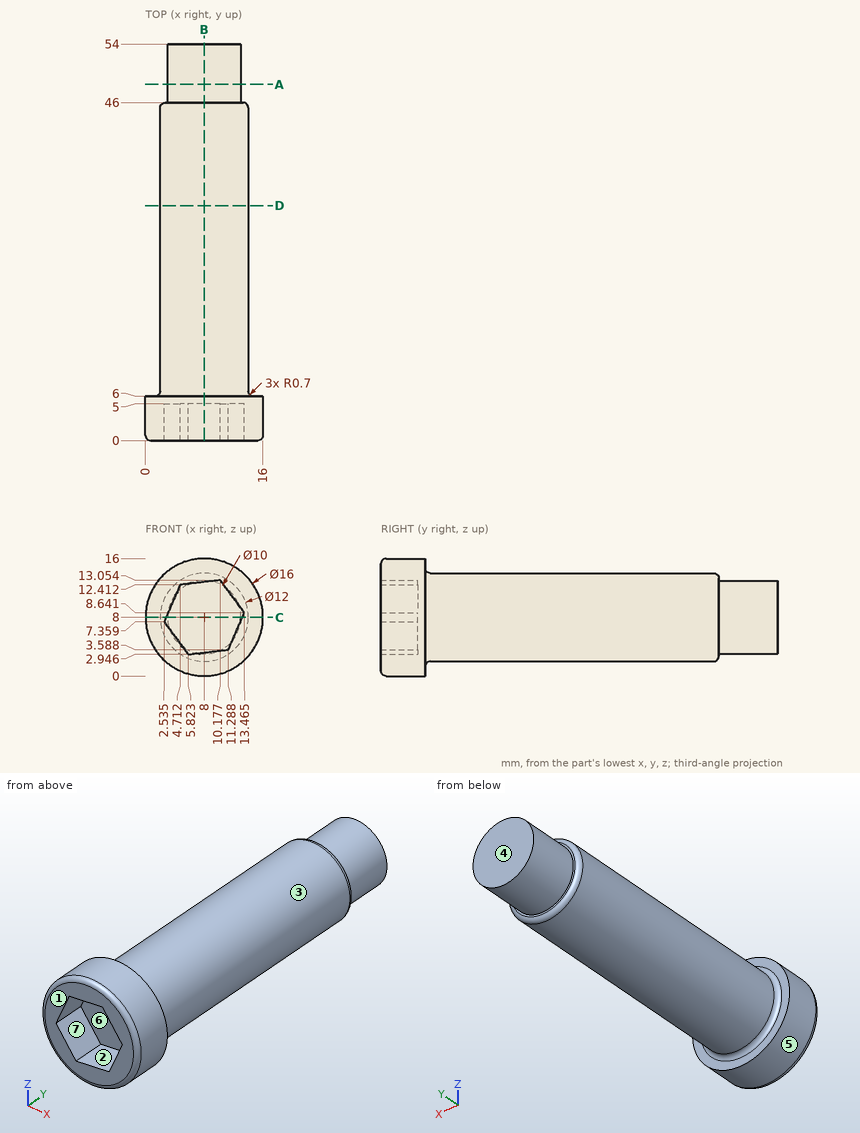
Could you check a few things on this drawing? It's one solid part, dimensions in mm from its lowest x, y, z. A direction names the side the tool comes from. Coordinates: 2 decimals unless noted, no trailing zeros. Order: outer loops, then holes, each group sorted by start corner. A loop starts at its lowest first (then second) coordinate and runs counter-clockwise, first axis right, second up. Notation, with made-up numbers: (39.25, 21.5) - (68.25, 21.5) arc R18 ccw to (68.25, 45.5) - close; hole circle Ø8 at (62.25, -11.5). An arc over 180 degrees is marked (long way). Answer as a JSON object with one key per item and string values. Group by question number.
Q1. Imagine slicing it at A-A (y = 48.5). Please give me the cut outline in (x, z).
Q2. Imagine slicing it at B-B (x = 8). Please give me the cut outline in (y, z).
Q3. On a 3-axis mill with a long thin cutter (end or side, diameter ignored), from which of +Z, -Z, +X, -X, +Y, -Y can I reach the whole of each face in a straight line? I mean the marked faces 1, 2 and 3. Say none if no direction works.
Q4. Imagine slicing it at D-D (y = 32). Please give me the cut outline in (x, z), and give its area (3 significant figures).
Q5. Will these pins go through, and if not, where does the flat tip stop? P1, Ø1.5, axis at y = 26, z = 8.5, coming from the -X side; P2, Ø2, axis at x = 10.5, y = 13.5, coming from the +Z side; P3, Ø3, axis at x = 3, y = 46.5, coming from the -Z side (1 decimal).
Q6. Imagine slicing it at C-C (z = 8). Please give me the cut outline in (x, y).
Q7. We'd pull the mould along X, two halves only. Please class the marked faces 4, 5, 6 and 7: +X half, -X half, draft (parallel to the pull), parting line (faces both ways), or undercut.
Q8. I need wall thicknesses on line 1 (Y direction, x = 5.75, z = 4.75); line 2 (Y direction, x = 12.25, z = 4.75); line 3 (Z direction, x = 7.75, y = 14) (1 decimal). Which ranges of each line are inside material? Lowest first, please. Write a range as from..to.
Determined:
{
 "1": {"outline": "circle Ø10 at (8, 8)"},
 "2": {"outline": "(0, 0.7) arc R0.7 ccw to (0.7, 0) - (6, 0) - (6, 1.3) arc R0.7 cw to (6.7, 2) - (45.3, 2) arc R0.7 ccw to (46, 2.7) - (46, 3) - (54, 3) - (54, 13) - (46, 13) - (46, 13.3) arc R0.7 ccw to (45.3, 14) - (6.7, 14) arc R0.7 cw to (6, 14.7) - (6, 16) - (0.7, 16) arc R0.7 ccw to (0, 15.3) - (0, 12.8) - (5, 12.8) - (5, 3.2) - (0, 3.2) - close"},
 "3": {"face 1": "+Z, -Z, +X, -X, -Y", "face 2": "-Y", "face 3": "+Y"},
 "4": {"outline": "circle Ø12 at (8, 8)", "area": "113 mm2"},
 "5": {"P1": "stops at x = 2", "P2": "stops at z = 13.81", "P3": "stops at z = 3.4"},
 "6": {"outline": "(0, 0.7) arc R0.7 ccw to (0.7, 0) - (2.81, 0) - (2.81, 5) - (13.19, 5) - (13.19, 0) - (15.3, 0) arc R0.7 ccw to (16, 0.7) - (16, 6) - (14.7, 6) arc R0.7 cw to (14, 6.7) - (14, 45.3) arc R0.7 ccw to (13.3, 46) - (13, 46) - (13, 54) - (3, 54) - (3, 46) - (2.7, 46) arc R0.7 ccw to (2, 45.3) - (2, 6.7) arc R0.7 cw to (1.3, 6) - (0, 6) - close"},
 "7": {"face 4": "draft", "face 5": "parting line", "face 6": "undercut", "face 7": "undercut"},
 "8": {"line 1": "y = 5..54", "line 2": "y = 0..46", "line 3": "z = 2..14"}
}
